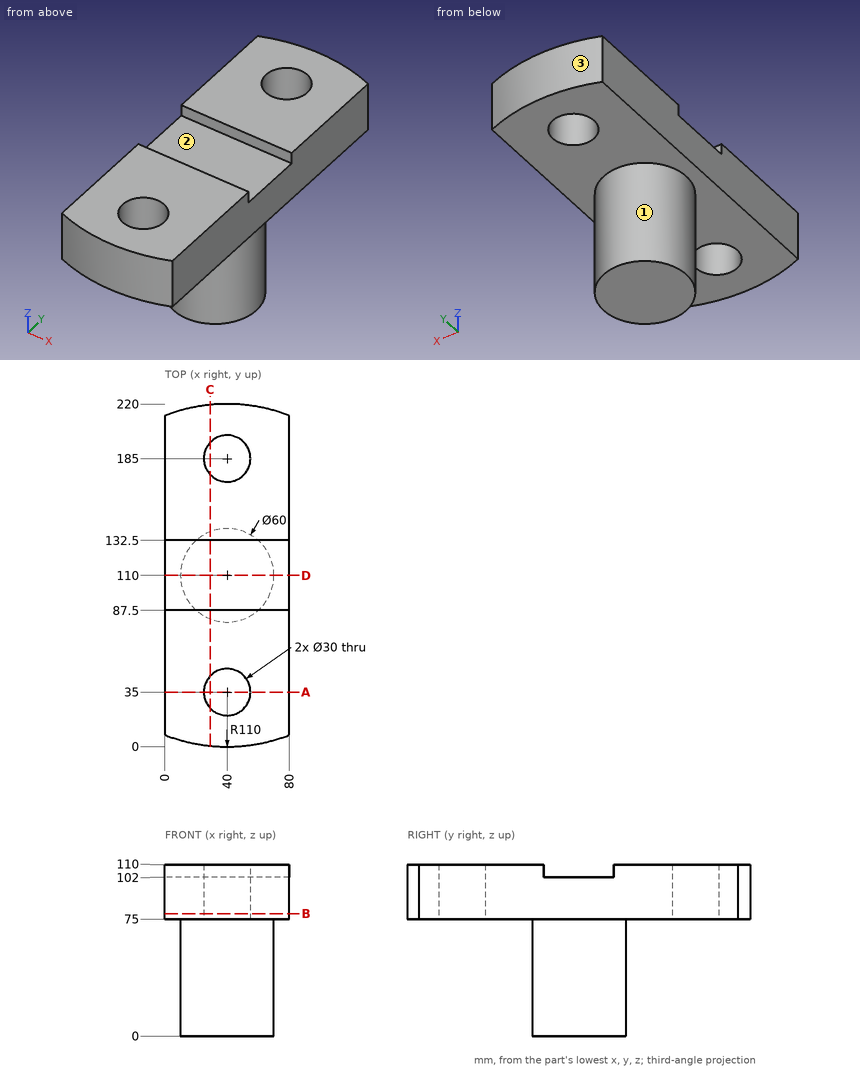
Drawing for the job (mm, zero at the part's lowest x, y, z). Coordinates: 2 decimals unless noted, no trailing zeros. Order: outer loops, then holes, each group sorted by start corner. A loop starts at its lowest first (then second) coordinate and runs counter-clockwise, first axis right, second up. Notation, with made-up numbers: (33.5, -38) - (72.5, -38) arc R34 ccw to (72.5, -1) - close; hole circle Ø11 at (-33.75, -25.5). An arc over 180 degrees is marked (long way). Use a Markdown table: item, result. Add a question column.
(1) Flat gauge pins, fed straight in: pin 1 (10 mm diameter, centred on y = 111.5, z = 34.5, fed in from -X); pin 2 (22.5 mm diameter, centred on x = 60, y = 113.5, fed in from +Z); pin 3 (1 mm diameter, centred on x = 8.5, y = 144, fed in from -Z); pin 4 (24 mm diameter, centred on x = 40, y = 185, fed in from +Z). Where does each tip first touch, or does it go through?
(2) Drill centre lines: line 1 along Y through (x, z) = (40, 98); line 2 along Z through (x, y) = (57.5, 194.5); line 3 along Z through (x, y) = (35.5, 120.5). Where is each one in solid material? Low to high. Write a range as [from, to].
(3) Pull direction Y, two halves, no side cores. Call the marked faces 1, 2 and 3: +Y half, -Y half, draft (parallel to the pull), parting line (faces both ways), or undercut.
(4) Saw through at B-B (z = 78.5). Give the cut face in (x, y), then the cut area to 3 significant figures.
(5) Saw through at A-A (y = 35). Give the cut face in (x, z), then the cut area to 3 significant figures.
(6) Saw through at C-C (x = 29). Give the cut face in (y, z).
(7) Saw through at D-D (y = 110). Give the cut face in (x, z).
Solved:
| question | item | result |
|---|---|---|
| 1 | pin 1 | stops at x = 10 |
| 1 | pin 2 | stops at z = 102 |
| 1 | pin 3 | stops at z = 75 |
| 1 | pin 4 | passes through |
| 2 | line 1 | y = [0, 20], [50, 170], [200, 220] |
| 2 | line 2 | z = [75, 110] |
| 2 | line 3 | z = [0, 102] |
| 3 | face 1 | parting line |
| 3 | face 2 | undercut |
| 3 | face 3 | +Y half |
| 4 | outline | (0, 7.53) arc R110 ccw to (80, 7.53) - (80, 212.47) arc R110 ccw to (0, 212.47) - close; hole circle Ø30 at (40, 35); hole circle Ø30 at (40, 185) |
| 4 | area | 15,800 mm² |
| 5 | outline | (0, 75) - (25, 75) - (25, 110) - (0, 110) - close; (55, 75) - (80, 75) - (80, 110) - (55, 110) - close |
| 5 | area | 1,750 mm² |
| 6 | outline | (0.55, 75) - (24.8, 75) - (24.8, 110) - (0.55, 110) - close; (45.2, 75) - (82.09, 75) - (82.09, 0) - (137.91, 0) - (137.91, 75) - (174.8, 75) - (174.8, 110) - (132.5, 110) - (132.5, 102) - (87.5, 102) - (87.5, 110) - (45.2, 110) - close; (195.2, 75) - (219.45, 75) - (219.45, 110) - (195.2, 110) - close |
| 7 | outline | (0, 75) - (10, 75) - (10, 0) - (70, 0) - (70, 75) - (80, 75) - (80, 102) - (0, 102) - close |
